Source: CAD feature listing. Evaluate the final solid. Frame: model axes, mm. A direction names the side the tool comes from. Coordinates: 2 decimals unless noted, no trailing zeros. Order: outer loops, then holes, each group sorted by start corner. A loop starts at its lowest first (then second) coordinate and runs counter-clockwise, first axis right, second up.
```python
from build123d import *

# Parameters (mm, degrees)
F1_DEPTH = 50
F2_W     = 88
F2_H     = 119
F3_DEPTH = 100.001
F4_R     = 5
F5_DEPTH = 88
F6_R     = 25
F7_DEPTH = 10
F8_R     = 75
F9_DEPTH = 25


with BuildPart() as f1:
    # F0 (on Right) → F1 (new body, symmetric)
    with BuildSketch(Plane.YZ):
        Polygon((0, -125), (0, 0), (-100, 0), (-100, -50), (-30, -125), align=None)
    extrude(amount=F1_DEPTH, both=True)

    # F2 (on face) → F3 (cut, through all)
    with BuildSketch(Plane(origin=(0, 0, 0), x_dir=(-1, 0, 0), z_dir=(0, 1, 0))):
        with Locations((0, -65.5)):
            Rectangle(F2_W, F2_H)
    extrude(amount=-F3_DEPTH, mode=Mode.SUBTRACT)

    # F4 (on face) → F5 (join, through all)
    with BuildSketch(Plane(origin=(44, 0, 0), x_dir=(0, -1, 0), z_dir=(-1, 0, 0))):
        with Locations((15, -110)):
            Circle(F4_R)
    extrude(amount=F5_DEPTH)

    # F6 (on face) → F7 (join)
    with BuildSketch(Plane.XY):
        with Locations((0, -50)):
            Circle(F6_R)
    extrude(amount=F7_DEPTH)

    # F8 (on Right) → F9 (join, symmetric)
    with BuildSketch(Plane.YZ):
        with Locations((-15, -110)):
            Circle(F8_R)
    extrude(amount=F9_DEPTH, both=True)


solid = f1.part
```
1. Access query for faces 4 (the flat face through (47.042, -65.49, -86.975)), 5 (the flat face through (-46.958, -65.49, -86.975)), 6 (the flat face through (47, -15, -125)), 7 (the cylindrical face through (-34.37, -19.77, -108.5)). Directions: +Z, -Z, +X, -X, +Y, -Y. A direction counts if a zero-diameter tool reaches every point of the face in a straight line with its end or side. Return the directions, or none.
2. Section query A-A, the plane y = -15. Output: boundary loops of the cut face in (x, z), plus the area to 3 significant figures.
3. Section query D-D, the plane y = -50. Output: boundary loops of the cut face in (x, z), plus the area to 3 significant figures.
4. Section query C-C, the plane z = -22. Output: boundary loops of the cut face in (x, y).
5. Section query B-B, the plane x = 14. Output: boundary loops of the cut face in (y, z), plus the area to 3 significant figures.
6. Material intervals for line 1 along X through (y, z) = (-37.5, -69); line 2 along X through (y, z) = (-45, -16); line 3 along X through (y, z) = (-55, -132.5), sorted ascending.
7. Draft query along X for faces 1 (the flat face through (50, -40, -48)), 2 (the flat face through (-47, -15, -125)), 3 (the flat face through (-44, -38, -53)). Return one class per face: +X half, -X half, draft (parallel to the pull), parting line (faces both ways), or undercut.
8. Contact query for flat-ended pins moving along their axis: P1, Ø3, axis at x = 47, y = -12, coming from the -Z side; P2, Ø5, axis at x = -17.5, y = -4.5, coming from the +Z side; P3, Ø6, axis at x = -24.5, z = -109, coming from the -Y side. Output: stop coordinate, or through.
Answer key:
1. face 4: -Z, +X, -Y
1. face 5: -Z, -X, -Y
1. face 6: -Z, +X, +Y, -Y
1. face 7: none
2. outline: (-50, -125) - (-44, -125) - (-44, -115) - (-25, -115) - (-25, -185) - (25, -185) - (25, -115) - (44, -115) - (44, -125) - (50, -125) - (50, 0) - (-50, 0) - close; hole (-44, -105) - (-25, -105) - (-25, -35) - (25, -35) - (25, -105) - (44, -105) - (44, -6) - (-44, -6) - close
2. area: 9,910 mm2
3. outline: (-50, -103.57) - (-44, -103.57) - (-44, -6) - (44, -6) - (44, -103.57) - (50, -103.57) - (50, 0) - (25, 0) - (25, 10) - (-25, 10) - (-25, 0) - (-50, 0) - close; (-25, -176.33) - (25, -176.33) - (25, -43.67) - (-25, -43.67) - close
3. area: 8,900 mm2
4. outline: (-50, -100) - (-44, -100) - (-44, 0) - (-50, 0) - close; (44, -100) - (50, -100) - (50, 0) - (44, 0) - close
5. outline: (-100, -6) - (0, -6) - (0, 0) - (-29.29, 0) - (-29.29, 10) - (-70.71, 10) - (-70.71, 0) - (-100, 0) - close; circle Ø150 at (-15, -110)
5. area: 18,700 mm2
6. line 1: x = -50 to -44, -25 to 25, 44 to 50
6. line 2: x = -50 to -44, 44 to 50
6. line 3: x = -25 to 25
7. face 1: +X half
7. face 2: draft
7. face 3: undercut
8. P1: stops at z = -125
8. P2: stops at z = 0
8. P3: stops at y = -90
